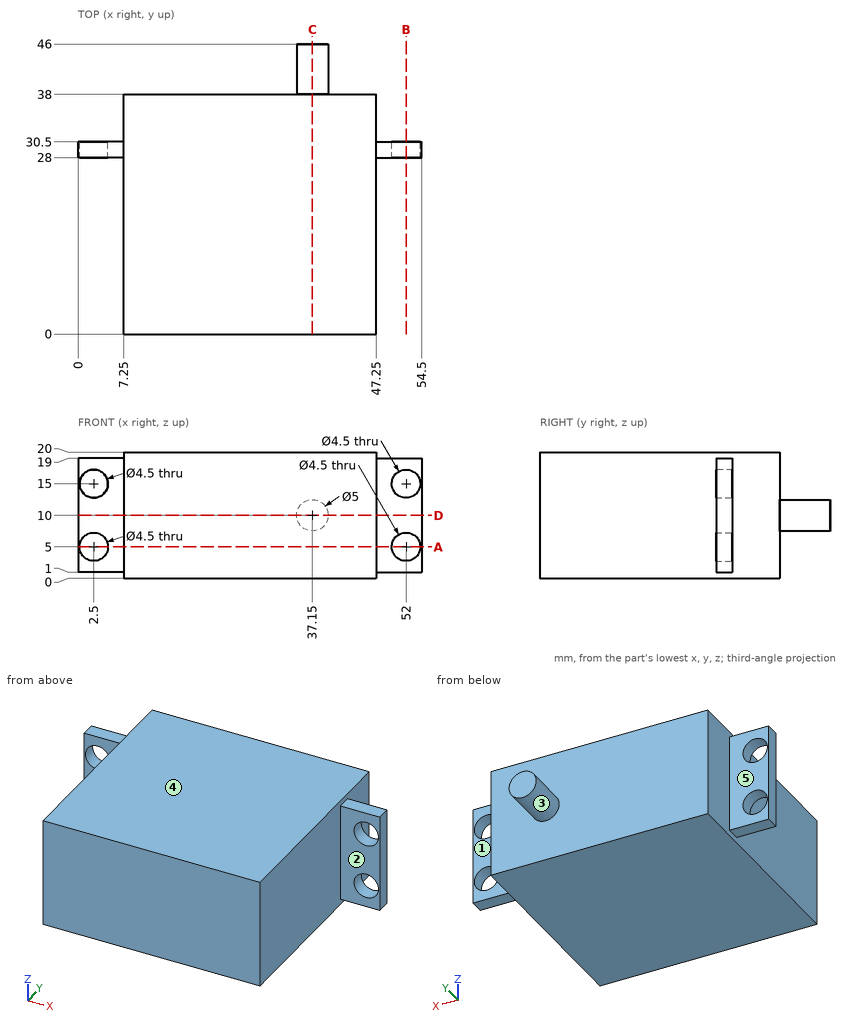
Geometry check sheet. Reference: drawing and pictorial views, mm from the part's lowest x, y, z. A direction names the side the tool comes from. Coordinates: 2 decimals unless noted, no trailing zeros. Write each loop counter-clockwise with the first axis right and the second up, starting at its lowest first coordinate (ties: lowest second). Pieces come first, ordered by that corner, then holes.
Item 1: Cross-section at A-A on z = 5. Record the boundary of the cut face in (x, y), then the cut area to 3 significant figures.
Numbers:
outline: (0, 28) - (0.25, 28) - (0.25, 30.5) - (0, 30.5) - close; (4.75, 28) - (7.25, 28) - (7.25, 0) - (47.25, 0) - (47.25, 28) - (49.75, 28) - (49.75, 30.5) - (47.25, 30.5) - (47.25, 38) - (7.25, 38) - (7.25, 30.5) - (4.75, 30.5) - close; (54.25, 28) - (54.5, 28) - (54.5, 30.5) - (54.25, 30.5) - close
area: 1,530 mm2
Item 2: Depth check by flat-ended pin: pin 1 Ø6 at (x, z) = (52, 5) entering from -Y; pin 2 Ø4 at (y, z) = (16.5, 2.5) entering from +X; pin 3 Ø8 at (x, z) = (2.5, 13) entering from +Y; pin 4 Ø4 at (x, z) = (2.5, 15) entering from -Y. Enter the tip coordinate at first touch or a pass-through.
Numbers:
pin 1: stops at y = 28
pin 2: stops at x = 47.25
pin 3: stops at y = 30.5
pin 4: passes through
Item 3: Cross-section at D-D on z = 10. Record the boundary of the cut face in (x, y), then the cut area to 3 significant figures.
Numbers:
outline: (0, 28) - (7.25, 28) - (7.25, 0) - (47.25, 0) - (47.25, 28) - (54.5, 28) - (54.5, 30.5) - (47.25, 30.5) - (47.25, 38) - (39.65, 38) - (39.65, 46) - (34.65, 46) - (34.65, 38) - (7.25, 38) - (7.25, 30.5) - (0, 30.5) - close
area: 1,600 mm2
Item 4: Access from +Z, -Z, +X, -X, +Y, -Y to the whole of each face (thin tool, end or side, straight path). Record for the marked faces 1, 2, 3, 4 and 5.
Numbers:
face 1: +Z, -Z, +X, +Y
face 2: +Z, -Z, +X, -Y
face 3: +Y
face 4: +Z, +X, -X, +Y, -Y
face 5: +Z, -Z, -X, +Y
Item 5: Scan lines: probe 1 along X at (y, z) = (29.6, 5); probe 2 along Y at (x, z) = (20, 15.5); probe 3 along Z at (x, y) = (2, 29). Record each from-to range of solid material in increasing order.
Numbers:
probe 1: x = 0 to 0.25, 4.75 to 49.75, 54.25 to 54.5
probe 2: y = 0 to 38
probe 3: z = 1 to 2.81, 7.19 to 12.81, 17.19 to 19
Item 6: Cross-section at C-C on x = 37.15. Record the boundary of the cut face in (y, z), then the cut area to 3 significant figures.
Numbers:
outline: (0, 0) - (38, 0) - (38, 7.5) - (46, 7.5) - (46, 12.5) - (38, 12.5) - (38, 20) - (0, 20) - close
area: 800 mm2
Item 7: Cross-section at B-B on x = 52. Record the boundary of the cut face in (y, z).
Numbers:
outline: (28, 1) - (30.5, 1) - (30.5, 2.75) - (28, 2.75) - close; (28, 7.25) - (30.5, 7.25) - (30.5, 12.75) - (28, 12.75) - close; (28, 17.25) - (30.5, 17.25) - (30.5, 19) - (28, 19) - close
